For this review, take the finished solid that the model builds, in its own axes (mm). A direction names the side the tool comes from. Round coordinates to 2 decimals unless told otherwise and drop trailing zeros. Loops run counter-clockwise (first coordinate to the right, second up) from the corner with the lowest first, then second, coordinate; pieces in that order, holes last. Notation, with made-up numbers: (-3, 79.25) -> (50, 79.25) arc R22 ccw to (50, 95.25) -> close; hole circle Ø6 at (24, 72.5). An arc over 180 degrees is marked (long way). Use one line per item in the form item = value. Start each with the question number.
from build123d import *

# Parameters (mm, degrees)
BOSS_EXTRUDE1_DEPTH = 63.5
SKETCH4_R           = 1.27
CUT_EXTRUDE2_DEPTH  = 63.5
SKETCH6_R           = 12.7
CUT_EXTRUDE7_DEPTH  = 1.5875
SKETCH8_R           = 4.826
CUT_EXTRUDE8_DEPTH  = 1.5875


with BuildPart() as part:
    # Sketch2 → Boss-Extrude1 (new body)
    with BuildSketch(Plane.XY):
        Polygon((-18.314458333, 3.81), (20.828, 3.81), (20.828, -8.89), (17.526, -8.89), (17.526, 0), (-17.526, 0), (-17.526, -8.89), (-20.828, -8.89), (-20.828, 3.81), align=None)
    extrude(amount=BOSS_EXTRUDE1_DEPTH)

    # Sketch4 → Cut-Extrude2 (cut)
    with BuildSketch(Plane.XZ.offset(8.89)):
        with Locations((-19.177, 7.62)):
            Circle(SKETCH4_R)
        with Locations((-19.177, 55.88)):
            Circle(SKETCH4_R)
        with Locations((-19.177, 31.75)):
            Circle(SKETCH4_R)
    cut_extrude2 = extrude(amount=-CUT_EXTRUDE2_DEPTH, mode=Mode.SUBTRACT)

    # Mirror1: Cut-Extrude2 across plane
    add(cut_extrude2.mirror(Plane(origin=(0, 0, 0), x_dir=(0, 0, 1), z_dir=(1, 0, 0))), mode=Mode.SUBTRACT)

    # Sketch6 → Cut-Extrude7 (cut)
    with BuildSketch(Plane(origin=(0, 3.81, 0), x_dir=(1, 0, 0), z_dir=(0, 1, 0))):
        with Locations((0, -13.97)):
            Circle(SKETCH6_R)
    extrude(amount=-CUT_EXTRUDE7_DEPTH, mode=Mode.SUBTRACT)

    # Sketch8 → Cut-Extrude8 (cut)
    with BuildSketch(Plane(origin=(0, 2.2225, 0), x_dir=(1, 0, 0), z_dir=(0, 1, 0))):
        with Locations((0, -13.97)):
            Circle(SKETCH8_R)
    extrude(amount=-CUT_EXTRUDE8_DEPTH, mode=Mode.SUBTRACT)


solid = part.part
Item 1: Draft analysis for pull direction X (two halves, no side actions). For faces 4 (the flat face through (20.828, -2, 31)), 5 (the flat face through (-20.828, -3, 31)), 6 (the cylindrical face through (18.004, -2.629, 31.264)), 7 (the flat face through (0.3, 0.4, 63.5)), state which applies: +X half, -X half, draft (parallel to the pull), parting line (faces both ways), or undercut.
Item 2: Machinability: for faces 1 (the flat face through (17.526, -5, 31)), 2 (the cylindrical face through (5.86, 3.027, 25.237)), 3 (the cylindrical face through (18.591, -2.629, 54.753)), which of the approach directions +Z, -Z, +X, -X, +Y, -Y give a long, thin tool a straight path to every point of the face, cutting with its end or side? Answer none if there is none.
Item 3: For P1, Ø6, axis at x = -13.5, z = 18.5, coming from the -Y side; P2, Ø1.5, axis at x = 7, z = 22, coming from the +Y side; P3, Ø3, axis at x = 2, z = 12.5, coming from the +Y side (3 decimals), all flat-tipped, find the tip position at first contact; note any pin that passes through.
Item 4: Take a section at A-A on y = -3.75. Give the boundary of the cut face in (x, z), plus the area to 3 significant figures.
Item 5: Take a section at B-B on z = 31.75. Give the boundary of the cut face in (x, y), plus the area to 3 significant figures.
Item 6: Wall thickness on line 1 (Z direction, x = 0, y = 1.1); line 2 (X direction, y = 3.1, z = 13.97); line 3 (X direction, y = -4.25, z = 20): over which ranges is each line inside the solid? List them lowest first.
Item 7: Take a section at D-D on x = 0. Give the boundary of the cut face in (y, z) (1 decimal), plus the area to 3 significant figures.
Item 8: Take a section at C-C on y = 1.5. Give the boundary of the cut face in (x, z).
Results:
q1.face_4 = +X half
q1.face_5 = -X half
q1.face_6 = undercut
q1.face_7 = draft
q2.face_1 = +Z, -Z, -Y
q2.face_2 = +Y
q2.face_3 = +Y, -Y
q3.P1 = 0
q3.P2 = 2.22
q3.P3 = 0.635
q4.outline = (-20.83, 0) -> (-17.53, 0) -> (-17.53, 63.5) -> (-20.83, 63.5) -> close; (17.53, 0) -> (20.83, 0) -> (20.83, 63.5) -> (17.53, 63.5) -> close; hole circle Ø2.54 at (-19.18, 7.62); hole circle Ø2.54 at (-19.18, 31.75); hole circle Ø2.54 at (-19.18, 55.88); hole circle Ø2.54 at (19.18, 7.62); hole circle Ø2.54 at (19.18, 31.75); hole circle Ø2.54 at (19.18, 55.88)
q4.area = 389 mm2
q5.outline = (-20.83, -8.89) -> (-20.45, -8.89) -> (-20.45, 3.81) -> (-20.83, 3.81) -> close; (-17.91, -8.89) -> (-17.53, -8.89) -> (-17.53, 0) -> (17.53, 0) -> (17.53, -8.89) -> (17.91, -8.89) -> (17.91, 3.81) -> (-17.91, 3.81) -> close; (20.45, -8.89) -> (20.83, -8.89) -> (20.83, 3.81) -> (20.45, 3.81) -> close
q5.area = 153 mm2
q6.line_1 = 0 to 9.14, 18.8 to 63.5
q6.line_2 = -20.83 to -12.7, 12.7 to 20.83
q6.line_3 = -20.83 to -17.53, 17.53 to 20.83
q7.outline = (0, 0) -> (3.8, 0) -> (3.8, 1.3) -> (2.2, 1.3) -> (2.2, 9.1) -> (0.6, 9.1) -> (0.6, 18.8) -> (2.2, 18.8) -> (2.2, 26.7) -> (3.8, 26.7) -> (3.8, 63.5) -> (0, 63.5) -> close
q7.area = 186 mm2
q8.outline = (-20.83, 0) -> (20.83, 0) -> (20.83, 63.5) -> (-20.83, 63.5) -> close; hole circle Ø2.54 at (-19.18, 7.62); hole circle Ø2.54 at (-19.18, 31.75); hole circle Ø2.54 at (-19.18, 55.88); hole circle Ø9.65 at (0, 13.97); hole circle Ø2.54 at (19.18, 7.62); hole circle Ø2.54 at (19.18, 31.75); hole circle Ø2.54 at (19.18, 55.88)
